Build history of the part. All positions in model axes, mm. A direction names the side the tool comes from. Round coordinates to 2 decimals unless told otherwise and drop trailing zeros. Loops run counter-clockwise (first coordinate to the right, second up) from the corner with the lowest first, then second, coordinate; pieces in that order, holes last. Notation, with made-up numbers: (28, -22.5) - (73, -22.5) arc R24 cw to (73, 8.5) - close; hole circle Ø3 at (58, 50). An arc over 180 degrees is marked (long way). Use a Markdown table: item, result.
from build123d import *

# Parameters (mm, degrees)
BOSS_EXTRUDE1_START = 0.15
SKETCH1_W           = 30
SKETCH1_H           = 10
SKETCH1_W_2         = 2.25
BOSS_EXTRUDE1_DEPTH = 2
SKETCH2_W           = 2
SKETCH2_H           = 10
BOSS_EXTRUDE2_DEPTH = 28.15
SKETCH3_W           = 2
SKETCH3_H           = 10
BOSS_EXTRUDE3_DEPTH = 10
FILLET1_R           = 2
CUT_EXTRUDE1_START  = -2
SKETCH4_R           = 1.5
CUT_EXTRUDE1_DEPTH  = 29.15


with BuildPart() as part:
    # Sketch1 → Boss-Extrude1 (new body)
    with BuildSketch(Plane.XY.offset(BOSS_EXTRUDE1_START)):
        with Locations((0, 5.545087163)):
            Rectangle(SKETCH1_W, SKETCH1_H)
        with Locations((16.125, 5.545087163)):
            Rectangle(SKETCH1_W_2, SKETCH1_H)
        with Locations((-16.125, 5.545087163)):
            Rectangle(SKETCH1_W_2, SKETCH1_H)
    extrude(amount=BOSS_EXTRUDE1_DEPTH)

    # Sketch2 → Boss-Extrude2 (add)
    with BuildSketch(Plane.XY.offset(2.15)):
        with Locations((18.25, 5.545087163)):
            Rectangle(SKETCH2_W, SKETCH2_H)
        with Locations((-18.25, 5.545087163)):
            Rectangle(SKETCH2_W, SKETCH2_H)
    extrude(amount=-BOSS_EXTRUDE2_DEPTH)

    # Sketch3 → Boss-Extrude3 (add)
    with BuildSketch(Plane.ZY.offset(19.25)):
        with Locations((-25, 5.545087163)):
            Rectangle(SKETCH3_W, SKETCH3_H)
    boss_extrude3 = extrude(amount=BOSS_EXTRUDE3_DEPTH)

    # Mirror1: Boss-Extrude3 across plane
    add(boss_extrude3.mirror(Plane(origin=(0, 0, 0), x_dir=(0, 0, 1), z_dir=(1, 0, 0))))

    # Fillet1
    fillet1_edges = [part.edges().sort_by_distance(p)[0] for p in [
        (19.25, 5.545087163, 2.15),
        (-19.25, 5.545087163, 2.15),
        (-19.25, 5.545087163, -24),
        (19.25, 5.545087163, -24),
    ]]
    fillet(fillet1_edges, radius=FILLET1_R)

    # Sketch4 → Cut-Extrude1 (cut)
    with BuildSketch(Plane.XY.offset(-24).offset(CUT_EXTRUDE1_START)):
        with Locations((-25.25, 5.545087163)):
            Circle(SKETCH4_R)
    cut_extrude1 = extrude(amount=CUT_EXTRUDE1_DEPTH, mode=Mode.SUBTRACT)

    # Mirror2: Cut-Extrude1 across plane
    add(cut_extrude1.mirror(Plane(origin=(0, 0, 0), x_dir=(0, 0, 1), z_dir=(1, 0, 0))), mode=Mode.SUBTRACT)


solid = part.part
Q1. Cut at A-A, the plane x = 25.25. List the corners of the cut face in (y, z).
Results found:
| item | result |
|---|---|
| outline | (0.55, -26) - (4.05, -26) - (4.05, -24) - (0.55, -24) - close; (7.05, -26) - (10.55, -26) - (10.55, -24) - (7.05, -24) - close |
Q2. Cut at C-C, the plane y = 6.5. List the corners of the cut face in (x, z).
Results found:
| item | result |
|---|---|
| outline | (-29.25, -26) - (-26.41, -26) - (-26.41, -24) - (-29.25, -24) - close; (-24.09, -26) - (-17.25, -26) - (-17.25, 0.15) - (17.25, 0.15) - (17.25, -26) - (24.09, -26) - (24.09, -24) - (21.25, -24) arc R2 cw to (19.25, -22) - (19.25, 0.15) arc R2 ccw to (17.25, 2.15) - (-17.25, 2.15) arc R2 ccw to (-19.25, 0.15) - (-19.25, -22) arc R2 cw to (-21.25, -24) - (-24.09, -24) - close; (26.41, -26) - (29.25, -26) - (29.25, -24) - (26.41, -24) - close |
Q3. Pull direction Y, two halves, no side cores. Call faces 4 (the face through (-4, 10.545, 1)), 5 (the face through (0, 6, 0.15)), 6 (the face through (-26.75, 5.61, -25.01)): pulls with the +Y half, pulls with the -Y half, needs draft (parallel to the pull), parting line crosses it, or undercut.
Results found:
| item | result |
|---|---|
| face 4 | pulls with the +Y half |
| face 5 | needs draft |
| face 6 | undercut |
Q4. Which spindle directions (+Z, -Z, +X, -X, +Y, -Y) get a long thin tool onto all of the face, cutting with end or side? Do faces 1 (the face through (19.25, 5, -11)), 2 (the face through (17.25, 5, -13)), 3 (the face through (-24, 4, -24)). Say none if no direction does.
Results found:
| item | result |
|---|---|
| face 1 | +Z, +X, +Y, -Y |
| face 2 | -Z, +Y, -Y |
| face 3 | +Z, -X, +Y, -Y |
Q5. Cut at D-D, the plane x = 15. List the corners of the cut face in (y, z).
Results found:
| item | result |
|---|---|
| outline | (0.55, 0.15) - (10.55, 0.15) - (10.55, 2.15) - (0.55, 2.15) - close |
Q6. Cut at B-B, the plane z = -11.5. List the corners of the cut face in (x, y), plus the area to 3 significant figures.
Results found:
| item | result |
|---|---|
| outline | (-19.25, 0.55) - (-17.25, 0.55) - (-17.25, 10.55) - (-19.25, 10.55) - close; (17.25, 0.55) - (19.25, 0.55) - (19.25, 10.55) - (17.25, 10.55) - close |
| area | 40.0 mm2 |
Q7. Drop flat-ended pins along their axis: pin 1 (2 mm diameter, centred on x = -16.5, z = -23, fed in from +Y); pin 2 (2 mm diameter, centred on y = 2.5, z = -19, fed in from -X); pin 3 (2 mm diameter, centred on x = -1.5, y = 3.5, fed in from -Z); pin 4 (3.5 mm diameter, centred on x = -25.25, y = 5.55, fed in from +Z). Give the stop position or say it passes through.
Results found:
| item | result |
|---|---|
| pin 1 | stops at y = 10.55 |
| pin 2 | stops at x = -19.25 |
| pin 3 | stops at z = 0.15 |
| pin 4 | stops at z = -24 |
Q8. Probe line 1 (X direction, y = 5.5, z = -24.5); line 2 (X direction, y = 8.5, z = -13.5); line 3 (Y direction, x = 25.25, z = -25.55). List the from-to ranges inside material, lowest first.
Results found:
| item | result |
|---|---|
| line 1 | x = -29.25 to -26.75, -23.75 to -17.25, 17.25 to 23.75, 26.75 to 29.25 |
| line 2 | x = -19.25 to -17.25, 17.25 to 19.25 |
| line 3 | y = 0.55 to 4.05, 7.05 to 10.55 |
